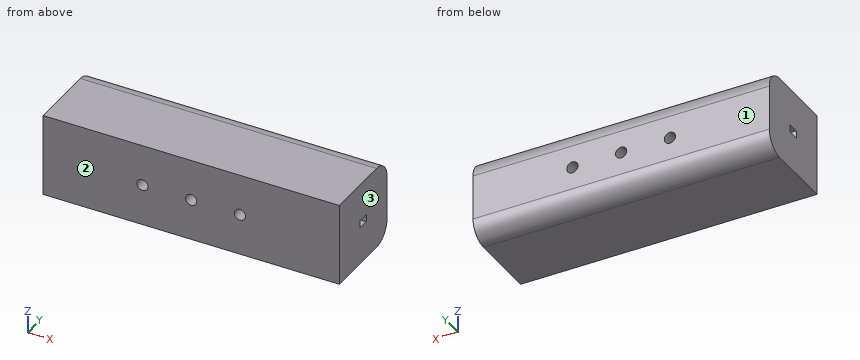
from build123d import *

# Parameters (mm, degrees)
EXTRUS_O_FINA1_DEPTH       = 39.5
EXTRUS_O_FINA1_DEPTH_BACK  = 39.5
CORTE_EXTRUS_O3_DEPTH      = 48.013295992
CORTE_EXTRUS_O3_DEPTH_BACK = 48.013295992
ESBO_O1_R                  = 1.5


with BuildPart() as part:
    # Esboço2 → Extrusão-Fina1 (new, two sides: drawn at the far end of the back side and taken through both)
    with BuildSketch(Plane(origin=(0, 0, 0), x_dir=(0, 0, -1), z_dir=(1, 0, 0)).offset(-EXTRUS_O_FINA1_DEPTH_BACK)):
        with BuildLine():
            Line((6, 23), (0, 23))
            Line((0, 23), (-6, 23))
            ThreePointArc((-6, 23), (-9.535533906, 21.535533906), (-11, 18))
            Line((-11, 18), (-11, 0))
            Line((-11, 0), (11, 0))
            Line((11, 0), (11, 18))
            ThreePointArc((11, 18), (9.535533906, 21.535533906), (6, 23))
        make_face()
        Polygon((1, 13), (0, 13), (-1, 13), (-1, 10), (1, 10), align=None, mode=Mode.SUBTRACT)
    extrude(amount=EXTRUS_O_FINA1_DEPTH + EXTRUS_O_FINA1_DEPTH_BACK)

    # Esboço1 → Corte-extrusão3 (cut, two sides: drawn at the far end of the back side and taken through both)
    with BuildSketch(Plane(origin=(0, 0, 0), x_dir=(1, 0, 0), z_dir=(0, 1, 0)).offset(-CORTE_EXTRUS_O3_DEPTH_BACK)):
        with Locations(Location((13, 0, 0), (0, 0, 270))):
            Circle(ESBO_O1_R)
        with Locations(Location((0, 0, 0), (0, 0, 270))):
            Circle(ESBO_O1_R)
        with Locations(Location((-13, 0, 0), (0, 0, 270))):
            Circle(ESBO_O1_R)
    extrude(amount=CORTE_EXTRUS_O3_DEPTH + CORTE_EXTRUS_O3_DEPTH_BACK, mode=Mode.SUBTRACT)


solid = part.part
The model under review builds one solid part; all positions refer to its coordinate system, in mm. Face numbers are marked on the shaded views. Round coordinates to 2 decimals unless told otherwise and drop trailing zeros. Write each loop counter-clockwise with the first axis right and the second up, starting at its lowest first coordinate (ties: lowest second). Pieces come first, ordered by that corner, then holes. Notation, with made-up numbers: (49, 70.25) -> (75, 70.25) arc R26 cw to (75, 96.25) -> close; hole circle Ø1 at (61.25, 51). An arc over 180 degrees is marked (long way). Answer as a JSON object with one key per item and string values.
1. We need section D-D on z = -9. State the section outline as (x, y) points.
Results found:
{"outline": "(-39.5, 0) -> (39.5, 0) -> (39.5, 22) -> (-39.5, 22) -> close"}
2. The part is to be moulded in two halves that separate along Y. For the marked faces 1, 2 and 3, say which applies: pulls with the +Y half, pulls with the -Y half, needs draft (parallel to the pull), parting line crosses it, or undercut.
Results found:
{"face 1": "pulls with the +Y half", "face 2": "pulls with the -Y half", "face 3": "needs draft"}
3. We need section B-B on z = 0. State how many separate pieces and enclosed holes the cut face has, and give its area (3 significant figures).
Results found:
{"separate pieces": "8", "enclosed holes": "0", "area": "1,400 mm^2"}
4. We need section A-A on x = -13. State the section outline as (y, z) points, and give its area (3 significant figures).
Results found:
{"outline": "(0, -11) -> (18, -11) arc R5 ccw to (23, -6) -> (23, -1.5) -> (0, -1.5) -> close; (0, 1.5) -> (23, 1.5) -> (23, 6) arc R5 ccw to (18, 11) -> (0, 11) -> close", "area": "426 mm^2"}
5. We need section C-C on x = -34. State the section outline as (y, z) points.
Results found:
{"outline": "(0, -11) -> (18, -11) arc R5 ccw to (23, -6) -> (23, 6) arc R5 ccw to (18, 11) -> (0, 11) -> close; hole (10, -1) -> (13, -1) -> (13, 1) -> (10, 1) -> close"}
6. Clearance check with flat-ended pins moving along their axes: pin 1 (2.5 mm diameter, centred on x = 0, z = 0, fed in from -Y); pin 2 (1.5 mm diameter, centred on x = -31.5, y = 19, fed in from -Z). State where each tip first meets the part, or that it passes through.
Results found:
{"pin 1": "passes through", "pin 2": "stops at z = -10.99"}
7. To check wall thickness, follow line 1 along X through (y, z) = (5, 0); line 2 along Z through (x, y) = (0, 13.25); line 3 along Z through (x, y) = (11.5, 10.75). State the ranges of each line that lie inside material, in increasing order.
Results found:
{"line 1": "x = -39.5 to -14.5, -11.5 to -1.5, 1.5 to 11.5, 14.5 to 39.5", "line 2": "z = -11 to -1.5, 1.5 to 11", "line 3": "z = -11 to -1, 1 to 11"}
